```python
from build123d import *

# Parameters (mm, degrees)
ESQUISSE1_W        = 15
ESQUISSE1_H        = 15
BOSS_EXTRU_1_DEPTH = 5
CONG_1_R           = 1
ESQUISSE2_R        = 1.5
BOSS_EXTRU_2_DEPTH = 0.3
CONG_2_R           = 1
ESQUISSE4_W        = 12
ESQUISSE4_H        = 12
BOSS_EXTRU_4_DEPTH = 2
CHANFREIN1_SIZE    = 1


with BuildPart() as part:
    # Esquisse1 → Boss.-Extru.1 (new body)
    with BuildSketch(Plane.XY):
        Rectangle(ESQUISSE1_W, ESQUISSE1_H)
    extrude(amount=BOSS_EXTRU_1_DEPTH)

    # Congé1
    cong_1_edges = [part.edges().sort_by_distance(p)[0] for p in [
        (7.5, -7.5, 2.5),
        (-7.5, -7.5, 2.5),
        (-7.5, 7.5, 2.5),
        (7.5, 7.5, 2.5),
    ]]
    fillet(cong_1_edges, radius=CONG_1_R)

    # Esquisse2 → Boss.-Extru.2 (add)
    with BuildSketch(Plane(origin=(0, 0, 0), x_dir=(-1, 0, 0), z_dir=(0, 0, -1))):
        with Locations((3.260921735, 0)):
            Circle(ESQUISSE2_R)
    extrude(amount=BOSS_EXTRU_2_DEPTH)

    # Congé2
    # the kernel refuses this fillet: 1 mm, written as the material it takes off along each edge
    with BuildSketch(Plane(origin=(-3.260921735, 0, -0.3), x_dir=(-1, 0, 0), z_dir=(0, -1, 0))) as cong_2_piece_1:
        with BuildLine():
            CenterArc((0.785857157, -1), CONG_2_R, 44.427004001, 45.572995999)
            Line((0.785857157, 0), (0.785857157, 0.02))
            Line((0.785857157, 0.02), (1.5, 0.02))
            Line((1.5, 0.02), (1.52, 0))
            ThreePointArc((1.52, 0), (1.52, -0.15), (1.514282857, -0.286))
            Line((1.514282857, -0.286), (1.5, -0.3))
        make_face()
    revolve(axis=Axis((-3.260921735, 0, -0.3), (0, 0, -1)), mode=Mode.SUBTRACT)

    # Esquisse4 → Boss.-Extru.4 (add)
    with BuildSketch(Plane.XY.offset(5)):
        Rectangle(ESQUISSE4_W, ESQUISSE4_H)
    extrude(amount=BOSS_EXTRU_4_DEPTH)

    # Chanfrein1
    chanfrein1_edges = [part.edges().sort_by_distance(p)[0] for p in [
        (6, -6, 6),
        (6, 6, 6),
        (-6, 6, 6),
        (-6, -6, 6),
    ]]
    chamfer(chanfrein1_edges, length=CHANFREIN1_SIZE)


solid = part.part
```
Design review of the part built by this model. Coordinates are the model's own, in mm. A direction names the side the tool comes from. Round coordinates to 2 decimals unless told otherwise and drop trailing zeros. Write each loop counter-clockwise with the first axis right and the second up, starting at its lowest first coordinate (ties: lowest second). Pieces come first, ordered by that corner, then holes.
Item 1: For faces 1 (the flat face through (0, 6, 6)), 2 (the flat face through (6, 0, 6)), 3 (the flat face through (5.5, -5.5, 6)), 4 (the flat face through (-5.5, 5.5, 6)), list the 3-axis set-ups (+Z, -Z, +X, -X, +Y, -Y) from which the entire face can be reached by the end or side of a thin tool; tool diameter is ignored.
Item 2: For probe 1 along Z at (x, y) = (0.5, -0.75); probe 2 along X at (y, z) = (4.25, 5.5), list the stretches that pass through material, from the lowest coordinate up.
Item 3: We need section C-C on y = 6.25. Write out the cut boundary in (x, z).
Item 4: We need section A-A on x = 2.75. Write out the cut boundary in (y, z).
Item 5: Clearance check with flat-ended pins moving along their axes: pin 1 Ø4.5 at (x, y) = (-3.5, 1.5) entering from -Z; pin 2 Ø2 at (y, z) = (0, 6.5) entering from -X; pin 3 Ø2 at (y, z) = (2, 6.5) entering from +X; pin 4 Ø0.6 at (x, z) = (-1.5, 6) entering from +Y. State where each tip first meets the part, or that it passes through.
Returned:
1. face 1: +Z, +X, -X, +Y
1. face 2: +Z, +X, +Y, -Y
1. face 3: +Z, +X, -Y
1. face 4: +Z, -X, +Y
2. probe 1: z = 0 to 7
2. probe 2: x = -6 to 6
3. outline: (-7.5, 0) - (7.5, 0) - (7.5, 5) - (-7.5, 5) - close
4. outline: (-7.5, 0) - (7.5, 0) - (7.5, 5) - (6, 5) - (6, 7) - (-6, 7) - (-6, 5) - (-7.5, 5) - close
5. pin 1: stops at z = -0.3
5. pin 2: stops at x = -6
5. pin 3: stops at x = 6
5. pin 4: stops at y = 6
